from build123d import *

# Parameters (mm, degrees)
F0_R            = 24.51608
F0_R_2          = 2.15265
F0_R_3          = 9.525
F1_DEPTH        = 5.08
F3_DEPTH        = 5.08
F3_COPIES_COUNT = 4
F4_R            = 0.762


# Not quite as in the source:
# - a pattern or mirror of a feature is missing from the dataset's text; its kind, count and spacing are read off the source's solid


with BuildPart() as f1:
    # F0 (on Top) → F1 (new body)
    with BuildSketch(Plane.XY):
        Circle(F0_R)
        with Locations((-11.7865906, -11.7865906)):
            Circle(F0_R_2, mode=Mode.SUBTRACT)
        with Locations((11.7865906, -11.7865906)):
            Circle(F0_R_2, mode=Mode.SUBTRACT)
        with Locations((-11.7865906, 11.7865906)):
            Circle(F0_R_2, mode=Mode.SUBTRACT)
        Circle(F0_R_3, mode=Mode.SUBTRACT)
        with Locations((11.7865906, 11.7865906)):
            Circle(F0_R_2, mode=Mode.SUBTRACT)
    extrude(amount=F1_DEPTH)

    # F2 (on face) → F3 (cut, through all)
    with BuildSketch(Plane.XY.offset(5.08)):
        with BuildLine():
            ThreePointArc((-12.5005198818, 17.2967828873), (-7.8454136559, 15.7030990397), (-6.2809895182, 11.0380782146))
            ThreePointArc((-6.2809895182, 11.0380782146), (0, 12.7), (6.2809895182, 11.0380782146))
            ThreePointArc((6.2809895182, 11.0380782146), (7.8454136559, 15.7030990397), (12.5005198818, 17.2967828873))
            ThreePointArc((12.5005198818, 17.2967828873), (0, 21.34108), (-12.5005198818, 17.2967828873))
        make_face()
    f3 = extrude(amount=-F3_DEPTH, mode=Mode.SUBTRACT)

    # F3_copies: F3 ×4 about axis
    f3_copies_axis = Axis((0, 0, 0), (0, 0, 1))
    for i in range(1, F3_COPIES_COUNT):
        add(f3.rotate(f3_copies_axis, i * 360 / F3_COPIES_COUNT), mode=Mode.SUBTRACT)

    # F4
    f4_edges = [f1.edges().sort_by_distance(p)[0] for p in [
        (-12.50052, 17.296783, 2.54),
        (12.50052, 17.296783, 2.54),
        (-17.296783, 12.50052, 2.54),
        (-17.296783, -12.50052, 2.54),
        (-12.50052, -17.296783, 2.54),
        (12.50052, -17.296783, 2.54),
        (17.296783, -12.50052, 2.54),
        (17.296783, 12.50052, 2.54),
    ]]
    fillet(f4_edges, radius=F4_R)


solid = f1.part
Check sheet for the modelled part. Datum: model origin and axes. Units: mm. A direction names the side the tool comes from. Round coordinates to 2 decimals unless told otherwise and drop trailing zeros. Order: outer loops, then holes, each group sorted by start corner. A loop starts at its lowest first (then second) coordinate and runs counter-clockwise, first axis right, second up.
Q1. Scan lines: L1, parallel to Y at x = 0, z = 3 (3 decimals); L2, parallel to X at y = -5, z = 2.7; L3, parallel to X at y = -10, z = 3.1. Record each from-to range of solid material in increasing order.
Filled sheet:
L1: y = -24.516 to -21.341, -12.7 to -9.525, 9.525 to 12.7, 21.341 to 24.516
L2: x = -24 to -20.75, -11.67 to -8.11, 8.11 to 11.67, 20.75 to 24
L3: x = -22.38 to -18.85, -17.05 to -12.99, -10.59 to 10.59, 12.99 to 17.05, 18.85 to 22.38
Q2. Set-up check for faces 4 (the face through (-0.15, -21.34, 2.58)), 5 (the face through (11, 0, 5.08)): record each of +Z, -Z, +X, -X, +Y, -Y from which the full face is reachable in a straight line by a thin tool's end or side.
Filled sheet:
face 4: +Z, -Z
face 5: +Z, +X, -X, +Y, -Y
Q3. Cross-section at A-A, the plane y = 0. Enter the section's corners in (x, z) (3 decimals), plus the area to 3 significant figures.
Filled sheet:
outline: (-24.516, 0) - (-21.341, 0) - (-21.341, 5.08) - (-24.516, 5.08) - close; (-12.7, 0) - (-9.525, 0) - (-9.525, 5.08) - (-12.7, 5.08) - close; (9.525, 0) - (12.7, 0) - (12.7, 5.08) - (9.525, 5.08) - close; (21.341, 0) - (24.516, 0) - (24.516, 5.08) - (21.341, 5.08) - close
area: 64.5 mm2
Q4. Cross-section at B-B, the plane x = 20. Enter the section's corners in (y, z), plus the area to 3 significant figures.
Filled sheet:
outline: (-14.18, 0) - (-7.45, 0) - (-7.45, 5.08) - (-14.18, 5.08) - close; (7.45, 0) - (14.18, 0) - (14.18, 5.08) - (7.45, 5.08) - close
area: 68.4 mm2
Q5. Depth check by flat-ended pin: P1, Ø15, axis at x = 0, y = 0, coming from the +Z side; P2, Ø5, axis at x = -11.79, y = -11.79, coming from the +Z side; P3, Ø1, axis at x = -10.5, z = 2.5, coming from the -Y side. Enter the tip coordinate at first touch or a pass-through.
Filled sheet:
P1: passes through
P2: stops at z = 5.08
P3: stops at y = -22.38
Q6. Draft check along Y on faces 1 (the face through (-7.13, -14.82, 2.58)), 2 (the face through (11, 0, 0)), 3 (the face through (-3.192, 24.307, 2.504)). Enter one of: pulls with the +Y half, pulls with the -Y half, needs draft (parallel to the pull), parting line crosses it, or undercut.
Filled sheet:
face 1: undercut
face 2: needs draft
face 3: parting line crosses it
Q7. Cross-section at D-D, the plane z = 2.8. Give the number of separate pieces and of enclosed holes in the cut face, plus the area to 3 significant figures.
Filled sheet:
separate pieces: 1
enclosed holes: 9
area: 971 mm2
